Print and shaded views of the part. All mm, measured from the part's lowest x, y and z. Round coordinates to 2 decimals unless told otherwise and drop trailing zeros. Loops run counter-clockwise (first coordinate to the right, second up) from the corner with the lowest first, then second, coordinate; pieces in that order, holes last. Notation, with made-up numbers: (80.25, 15) - (94.25, 15) arc R10 ccw to (94.25, 24) - close; hole circle Ø5 at (19.25, 73.5). An arc over 180 degrees is marked (long way). Use one line per item in the form item = value. Start each with the question number.
Q1. Drill centre lines: line 1 (Z direction, x = 26.45, y = 13); line 2 (Y direction, x = 43, z = 15); line 3 (X direction, y = 6.5, z = 36.5). Where is each one in solid material? Low to high.
Q2. Pin check, flat tips, straight feed: pin 1 (4.5 mm diameter, centred on x = 37.67, z = 45.89, fed in from +Y); pin 2 (1.5 mm diameter, centred on x = 16, y = 14, fed in from +Z); pin 3 (3 mm diameter, centred on y = 11, z = 11.5, fed in from -X). Stop position of each tip, or through.
Q3. Mould opens along X. For the marked faces 1, 2 and 3 say: released by +X, released by -X, zero draft, split by the parting line, or undercut.
Q4. Saw through at B-B (y = 14.75). Give the cut face in (x, z).
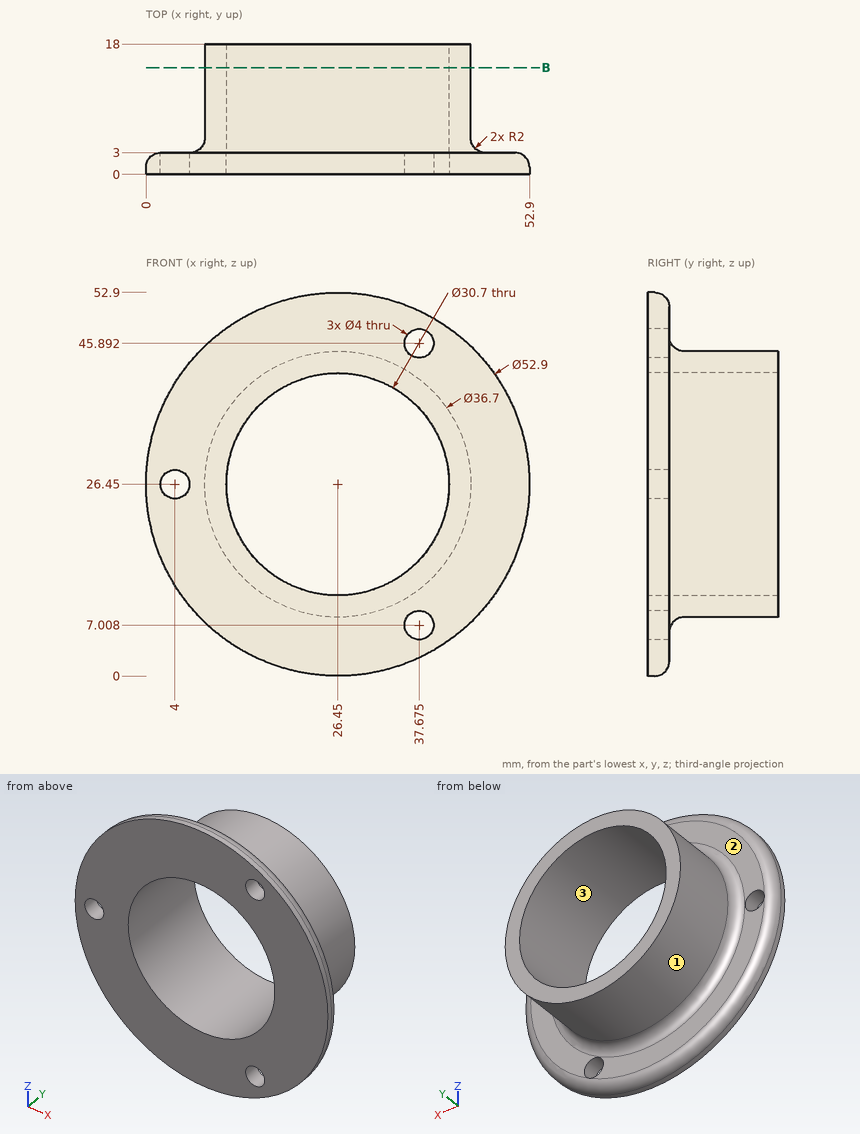
Report:
q1.line_1 = 8.1 to 11.1, 41.8 to 44.8
q1.line_2 = 0 to 3.01
q1.line_3 = 11.1 to 14.85, 38.05 to 41.8
q2.pin_1 = 3.01
q2.pin_2 = 42.03
q2.pin_3 = 13.97
q3.face_1 = split by the parting line
q3.face_2 = zero draft
q3.face_3 = undercut
q4.outline = circle Ø36.7 at (26.45, 26.45); hole circle Ø30.7 at (26.45, 26.45)
